Input: dimensioned drawing with shaded views. Units: mm. Origin: part minimum x, y, z. A direction names the side the tool comes from. Give positions to 0.01 mm unless a question says otherwise; leave off trailing zeros. Write each loop counter-clockwise with the first axis right and the second up, starting at its lowest first coordinate (ties: lowest second). Pieces come first, ordered by that corner, then holes. Notation, with made-up numbers: (-12.75, 84.25) -> (17.25, 84.25) arc R22 ccw to (17.25, 113.25) -> close; hole circle Ø9 at (-13, -5). An arc over 180 degrees is marked (long way). Answer as a JSON object with one key per item and string values. Group by question number.
(1) Draft query along X for the marked faces 4, 5, 6 and 7. Return one class per face: +X half, -X half, draft (parallel to the pull), parting line (faces both ways), or undercut.
(2) Section query C-C on z = 4.5. Output: boundary loops of the cut face in (x, y).
(3) Contact query for flat-ended pins moving along their axis: pin 1 Ø1 at (y, z) = (4.5, 3.5) entering from +X; pin 2 Ø5.5 at (x, z) = (13.5, 4.5) entering from -Y; pin 3 Ø3 at (x, z) = (13, 4.5) entering from -Y. Output: stop coordinate, or through.
(4) Section query D-D on y = 1.25. Output: boundary loops of the cut face in (x, z) (1 decimal).
(5) Section query B-B on z = 8. Output: boundary loops of the cut face in (x, y).
(6) Section query A-A on y = 4.25. Output: boundary loops of the cut face in (x, z).
(7) Set-up query: the marked faces 1, 2 and 3. Return all of +Z, -Z, +X, -X, +Y, -Y with unobstructed straight access to the full face (end or side cutting, diameter ignored); none if empty.
(8) Material intervals for probe 1 along X at (y, z) = (3.75, 1.5); probe 2 along Y at (x, z) = (15.75, 3); probe 3 along Z at (x, y) = (13.25, 6.25), sorted ascending.
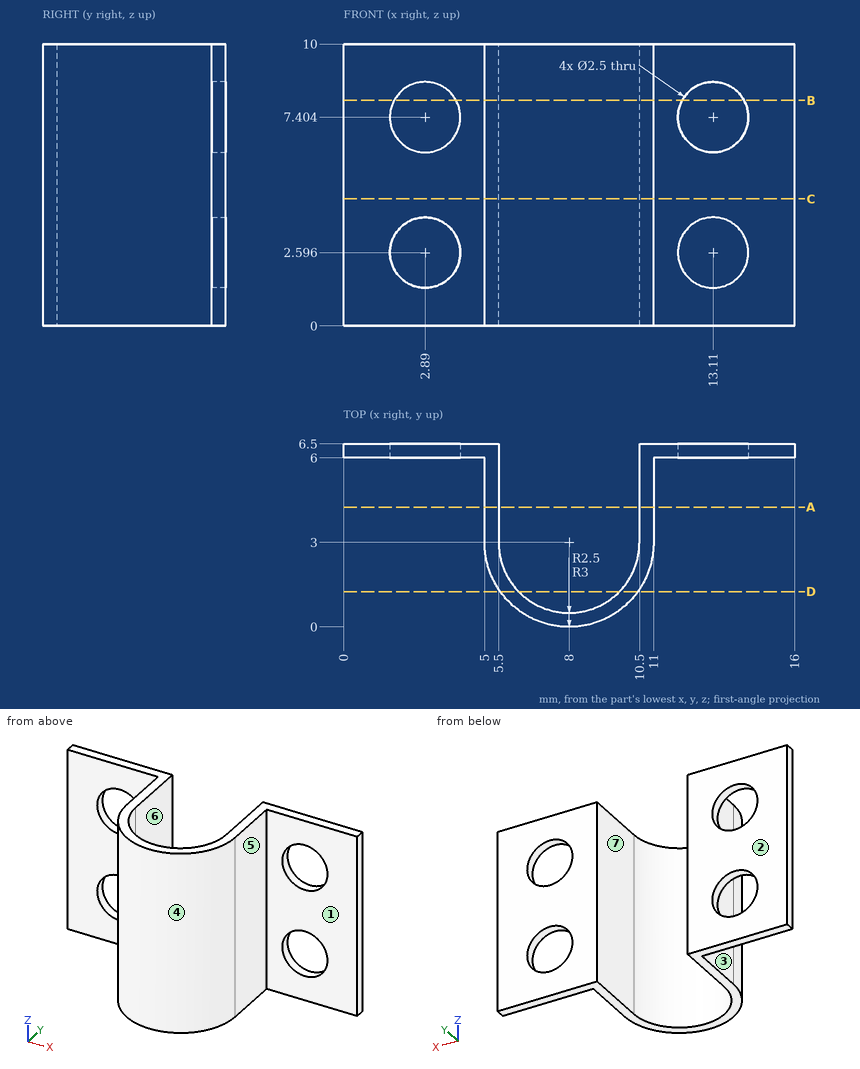
Answer list:
{
 "1": {"face 4": "parting line", "face 5": "+X half", "face 6": "undercut", "face 7": "undercut"},
 "2": {"outline": "(0, 6) -> (5, 6) -> (5, 3) arc R3 ccw to (11, 3) -> (11, 6) -> (16, 6) -> (16, 6.5) -> (10.5, 6.5) -> (10.5, 3) arc R2.5 cw to (5.5, 3) -> (5.5, 6.5) -> (0, 6.5) -> close"},
 "3": {"pin 1": "x = 11", "pin 2": "y = 1.8", "pin 3": "y = 6"},
 "4": {"outline": "(5.6, 0) -> (6.2, 0) -> (6.2, 10) -> (5.6, 10) -> close; (9.8, 0) -> (10.4, 0) -> (10.4, 10) -> (9.8, 10) -> close"},
 "5": {"outline": "(0, 6) -> (1.79, 6) -> (1.79, 6.5) -> (0, 6.5) -> close; (3.99, 6) -> (5, 6) -> (5, 3) arc R3 ccw to (11, 3) -> (11, 6) -> (12.01, 6) -> (12.01, 6.5) -> (10.5, 6.5) -> (10.5, 3) arc R2.5 cw to (5.5, 3) -> (5.5, 6.5) -> (3.99, 6.5) -> close; (14.21, 6) -> (16, 6) -> (16, 6.5) -> (14.21, 6.5) -> close"},
 "6": {"outline": "(5, 0) -> (5.5, 0) -> (5.5, 10) -> (5, 10) -> close; (10.5, 0) -> (11, 0) -> (11, 10) -> (10.5, 10) -> close"},
 "7": {"face 1": "+Z, -Z, +X, -Y", "face 2": "+Z, -Z, +X, -X, +Y", "face 3": "+Z, -Z, -X, -Y"},
 "8": {"probe 1": "5 to 5.5, 10.5 to 11", "probe 2": "6 to 6.5", "probe 3": "0 to 1.35, 3.84 to 6.16, 8.65 to 10"}
}
